Read the model definition and answer for the solid it produces. Units are mm, in the model's axes. A direction names the side the tool comes from. Round coordinates to 2 decimals unless told otherwise and drop trailing zeros. Order: outer loops, then holes, each group sorted by start corner. A loop starts at its lowest first (then second) coordinate and runs counter-clockwise, first axis right, second up. Notation, with made-up numbers: (76.5, 14.5) - (107.5, 14.5) arc R8 cw to (107.5, 26.5) - close; hole circle Ø4 at (26.25, -37). An arc over 180 degrees is marked (long way). Put each result on its own line as item: value. Start each with the question number.
Q1. Section A-A on y = -107 is taken. Give the vertices of the cut face in (x, z), then the cut area to 3 significant figures.
Q2. Section C-C on x = 152 is taken. Give the vertices of the cut face in (y, z).
Q3. Which of the six approach directions +Z, -Z, +X, -X, +Y, -Y give full straight-line access (tool end or side, diameter ignored) to faces 1 (the face through (200, 210, 417)), 2 (the face through (-210, -3, 270)), 3 (the face through (-84.26, 205.92, 356.2))?
Q4. Find the intervals of material crossed by line 1 along Y through (x, z) = (-130, 216.5); line 2 along X through (y, z) = (-131.5, 664); line 3 along Z through (x, y) = (119, -150), in increasing order. Write a range as from..to.
Q5. For a pull along Y with two mould halves and no side action, classify faces 4 (the face through (-3, -220, 407)), 5 (the face through (-79.56, -205.92, 370.17)), 6 (the face through (220, -3, 10)) as pulls with the +Y half, pulls with the -Y half, needs draft (parallel to the pull), parting line crosses it, or undercut.
Q6. Each of these flat-tipped pins is pushed along its axis until it touches: pin 1 Ø22 at (y, z) = (211, 274) entering from +X; pin 2 Ø8 at (x, y) = (174, 130) entering from +Z; pin 3 Ø6 at (x, y) = (-211, -91.5) entering from +Z. Where does it stop, or does it pass through?
Q7. Section D-D on z = 113 is taken. Give the vertices of the cut face in (x, y).
Q8. Section B-B on z = 360 is taken. Give the vertices of the cut face in (x, y).
from build123d import *

# Parameters (mm, degrees)
SKETCH1_W           = 440
SKETCH1_H           = 440
BOSS_EXTRUDE1_DEPTH = 20
SKETCH2_W           = 420
SKETCH2_H           = 20
BOSS_EXTRUDE2_DEPTH = 805
SKETCH3_W           = 20
SKETCH3_H           = 250
BOSS_EXTRUDE3_DEPTH = 400
SKETCH4_W           = 20
SKETCH4_H           = 250
BOSS_EXTRUDE4_DEPTH = 400
CUT_EXTRUDE1_DEPTH  = 12


with BuildPart() as part:
    # Sketch1 → Boss-Extrude1 (new body)
    with BuildSketch(Plane.XY):
        Rectangle(SKETCH1_W, SKETCH1_H)
    extrude(amount=BOSS_EXTRUDE1_DEPTH)

    # Sketch2 → Boss-Extrude2 (add)
    with BuildSketch(Plane.XY.offset(20)):
        with Locations((-10, -210)):
            Rectangle(SKETCH2_W, SKETCH2_H)
    boss_extrude2 = extrude(amount=BOSS_EXTRUDE2_DEPTH)

    # Sketch3 → Boss-Extrude3 (add)
    with BuildSketch(Plane(origin=(0, -200, 0), x_dir=(1, 0, 0), z_dir=(0, 1, 0))):
        with Locations((-210, -145)):
            Rectangle(SKETCH3_W, SKETCH3_H)
    extrude(amount=BOSS_EXTRUDE3_DEPTH)

    # Sketch4 → Boss-Extrude4 (add)
    with BuildSketch(Plane(origin=(0, -200, 0), x_dir=(1, 0, 0), z_dir=(0, 1, 0))):
        with Locations((-210, -670)):
            Rectangle(SKETCH4_W, SKETCH4_H)
    extrude(amount=BOSS_EXTRUDE4_DEPTH)

    # Sketch5 → Cut-Extrude1 (cut)
    with BuildSketch(Plane(origin=(0, -200, 0), x_dir=(1, 0, 0), z_dir=(0, 1, 0))):
        with BuildLine():
            ThreePointArc((-150, -705), (-77.574670949, -365.69256628), (127.077366481, -85.527424904))
            ThreePointArc((127.077366481, -85.527424904), (128.936250611, -84.394848326), (131.076875452, -84))
            Line((131.076875452, -84), (169.376524617, -84))
            ThreePointArc((169.376524617, -84), (170.504676767, -84.348554352), (171.239606574, -85.272727273))
            ThreePointArc((171.239606574, -85.272727273), (175.147542667, -87.43957679), (178, -84))
            Line((178, -84), (178, -74))
            Line((178, -74), (129.170663521, -74))
            ThreePointArc((129.170663521, -74), (125.25802282, -74.719375372), (121.857138002, -76.783410411))
            ThreePointArc((121.857138002, -76.783410411), (-86.307144971, -360.725571064), (-160, -705))
            Line((-160, -705), (-160, -780))
            ThreePointArc((-160, -780), (-155, -785), (-150, -780))
            Line((-150, -780), (-150, -705))
        make_face()
    cut_extrude1 = extrude(amount=-CUT_EXTRUDE1_DEPTH, mode=Mode.SUBTRACT)

    # Mirror1: Boss-Extrude2, Cut-Extrude1 across plane
    add(boss_extrude2.mirror(Plane.ZX))
    add(cut_extrude1.mirror(Plane.ZX), mode=Mode.SUBTRACT)


solid = part.part
Findings:
1. outline: (-220, 0) - (220, 0) - (220, 20) - (-200, 20) - (-200, 270) - (-220, 270) - close; (-220, 545) - (-200, 545) - (-200, 795) - (-220, 795) - close
1. area: 18,800 mm2
2. outline: (-220, 0) - (220, 0) - (220, 825) - (200, 825) - (200, 84) - (212, 84) - (212, 74) - (200, 74) - (200, 20) - (-200, 20) - (-200, 74) - (-212, 74) - (-212, 84) - (-200, 84) - (-200, 825) - (-220, 825) - close
3. face 1: +Z, +X, +Y, -Y
3. face 2: +X, -X
3. face 3: none
4. line 1: -220..-200, 200..220
4. line 2: -220..-200
4. line 3: 0..20
5. face 4: pulls with the -Y half
5. face 5: undercut
5. face 6: needs draft
6. pin 1: x = 200
6. pin 2: z = 20
6. pin 3: z = 795
7. outline: (-220, -220) - (200, -220) - (200, -200) - (97.81, -200) - (97.81, -212) - (83.65, -212) - (83.65, -200) - (-200, -200) - (-200, 200) - (83.65, 200) - (83.65, 212) - (97.81, 212) - (97.81, 200) - (200, 200) - (200, 220) - (-220, 220) - close
8. outline: (-220, -220) - (200, -220) - (200, -200) - (-75, -200) - (-75, -212) - (-85.98, -212) - (-85.98, -200) - (-220, -200) - close; (-220, 200) - (-85.98, 200) - (-85.98, 212) - (-75, 212) - (-75, 200) - (200, 200) - (200, 220) - (-220, 220) - close
